Verification items for this drawing (mm, ordinates from the low corner). Round coordinates to 2 decimals unless told otherwise and drop trailing zeros. Write each loop counter-clockwise with the first axis right and the second up, starting at its lowest first coordinate (ties: lowest second). Pieces come first, ordered by that corner, then holes. Notation, with made-up numbers: (24, -8) -> (42, -8) arc R22 ccw to (42, 11) -> close; hole circle Ø6 at (-34, 58). An arc over 180 degrees is marked (long way). One line per item, written item: value.
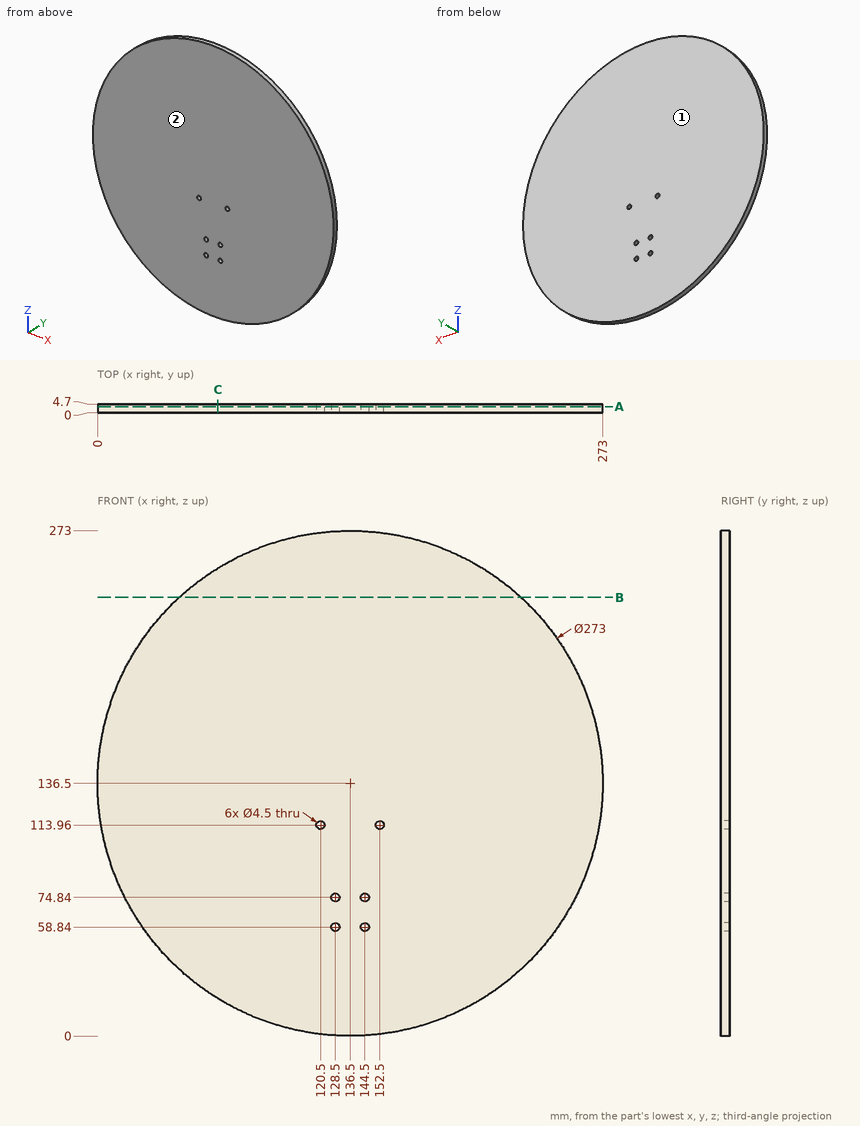
Item 1: Sectioned sample at C-C (x = 65). Enter the section's corners in (y, z), then the cut area to 3 significant figures.
Result set:
outline: (0, 20.22) -> (4.7, 20.22) -> (4.7, 252.78) -> (0, 252.78) -> close
area: 1,090 mm^2
Item 2: Sectioned sample at B-B (z = 237). Enter the section's corners in (x, y).
Result set:
outline: (44.13, 0) -> (228.87, 0) -> (228.87, 4.7) -> (44.13, 4.7) -> close
Item 3: Sectioned sample at A-A (y = 3.3). Enter the section's corners in (x, z).
Result set:
outline: circle Ø273 at (136.5, 136.5); hole circle Ø4.5 at (120.5, 113.96); hole circle Ø4.5 at (128.5, 58.84); hole circle Ø4.5 at (128.5, 74.84); hole circle Ø4.5 at (144.5, 58.84); hole circle Ø4.5 at (144.5, 74.84); hole circle Ø4.5 at (152.5, 113.96)
Item 4: Material ranges on line 1 along X through (y, z) = (2.6, 58.84); line 2 along X through (y, z) = (2.5, 74.84); line 3 along Z through (x, y) = (128.5, 2.85), recorded low to high.
Result set:
line 1: 24.25 to 126.25, 130.75 to 142.25, 146.75 to 248.75
line 2: 14.72 to 126.25, 130.75 to 142.25, 146.75 to 258.28
line 3: 0.23 to 56.59, 61.09 to 72.59, 77.09 to 272.77
Item 5: Depth check by flat-ended pin: pin 1 (1.5 mm diameter, centred on y = 2, z = 220.5, fed in from +X); pin 2 (1 mm diameter, centred on y = 3.5, z = 237, fed in from +X). Enter the tip coordinate at first touch or a pass-through.
Result set:
pin 1: x = 244.67
pin 2: x = 229.41
Item 6: Release check for a two-part mould opening along Y. For the marked faces 1 and 2 record: pulls with the +Y half, pulls with the -Y half, needs draft (parallel to the pull), parting line crosses it, or undercut.
Result set:
face 1: pulls with the +Y half
face 2: pulls with the -Y half
